For this review, take the finished solid that the model builds, in its own axes (mm). A direction names the side the tool comes from. Give positions to 0.01 mm unless a question says otherwise; leave off trailing zeros. Write each loop counter-clockwise with the first axis right and the second up, starting at its lowest first coordinate (ties: lowest second). Pieces come first, ordered by that corner, then holes. Notation, with made-up numbers: (26.5, -24.5) -> (53.5, -24.5) arc R20 cw to (53.5, -18.5) -> close; hole circle Ø5 at (58, -33). An arc over 180 degrees is marked (long way). Return JSON: item names as keys, results as strings.
from build123d import *

# Parameters (mm, degrees)
CROQUIS2_R            = 2
CORTAR_EXTRUIR1_DEPTH = 10
REDONDEO1_R           = 3


with BuildPart() as part:
    # Croquis1 → Revolución1 (revolve)
    with BuildSketch(Plane.XY, mode=Mode.PRIVATE) as revoluci_n1_sk:
        Polygon((0, 0), (2, 0), (2, 12), (7, 12), (7, 20), (8.25, 20), (8.25, 32.5), (0, 32.5), align=None)
    revolve(revoluci_n1_sk.sketch.rotate(Axis((0, 32.5, 0), (0, -1, 0)), 90), axis=Axis((0, 32.5, 0), (0, -1, 0)))

    # Croquis2 → Cortar-Extruir1 (cut)
    with BuildSketch(Plane(origin=(0, 32.5, 0), x_dir=(1, 0, 0), z_dir=(0, 1, 0))):
        with Locations(Location((0, 0, 0), (0, 0, 270))):
            Circle(CROQUIS2_R)
    extrude(amount=-CORTAR_EXTRUIR1_DEPTH, mode=Mode.SUBTRACT)

    # Redondeo1
    redondeo1_edges = [part.edges().sort_by_distance(p)[0] for p in [
        (0, 32.5, -8.25),
    ]]
    fillet(redondeo1_edges, radius=REDONDEO1_R)


solid = part.part
1. Add section D-D, the plane y = 9.5. State the section outline as (x, z) points.
Results found:
{"outline": "circle Ø4 at (0, 0)"}
2. For pin 1 (4 mm diameter, centred on x = 0.5, y = 20, fed in from +Z); pin 2 (5 mm diameter, centred on y = 23.5, z = -3, fed in from -X); pin 3 (5 mm diameter, centred on y = 20.5, z = 3, fed in from +X); pin 4 (4 mm diameter, centred on y = 17.5, z = -2.5, fed in from +X), all flat-tipped, find the tip position at first contact; note any pin that passes through.
Results found:
{"pin 1": "stops at z = 8.25", "pin 2": "stops at x = -8.23", "pin 3": "stops at x = 8.23", "pin 4": "stops at x = 6.98"}
3. Add section B-B, the plane y = 27. State the section outline as (x, z) points, plus the area to 3 significant figures.
Results found:
{"outline": "circle Ø16.5 at (0, 0); hole circle Ø4 at (0, 0)", "area": "201 mm²"}
4. For faces 1 (the cylindrical face through (6.21, 16.06, 3.23)), 2 (the flat face through (0, 0, 0)), list the 3-axis set-ups (+Z, -Z, +X, -X, +Y, -Y) from which the entire face can be reached by the end or side of a thin tool; tool diameter is ignored.
Results found:
{"face 1": "-Y", "face 2": "+Z, -Z, +X, -X, -Y"}
5. The part is to be moulded in two halves that separate along X. For faces 3 (the cylindrical face through (2, 6, 0)), 4 (the flat face through (0, 22.5, 0)), 5 (the flat face through (-0.1, 32.5, 2.3)), 6 (the cylindrical face through (-2, 28, 0)), say which applies: +X half, -X half, draft (parallel to the pull), parting line (faces both ways), or undercut.
Results found:
{"face 3": "parting line", "face 4": "undercut", "face 5": "draft", "face 6": "undercut"}
6. Add section A-A, the plane z = 0. State the section outline as (x, y) points.
Results found:
{"outline": "(-8.25, 20) -> (-7, 20) -> (-7, 12) -> (-2, 12) -> (-2, 0) -> (2, 0) -> (2, 12) -> (7, 12) -> (7, 20) -> (8.25, 20) -> (8.25, 29.5) arc R3 ccw to (5.25, 32.5) -> (2, 32.5) -> (2, 22.5) -> (-2, 22.5) -> (-2, 32.5) -> (-5.25, 32.5) arc R3 ccw to (-8.25, 29.5) -> close"}
7. To check wall thickness, follow probe 1 along X at (y, z) = (25.5, 0); probe 2 along Y at (x, z) = (-3.25, -3); probe 3 along X at (y, z) = (24.5, 0.75). State the ranges of each line that lie inside material, in increasing order.
Results found:
{"probe 1": "x = -8.25 to -2, 2 to 8.25", "probe 2": "y = 12 to 32.5", "probe 3": "x = -8.22 to -1.85, 1.85 to 8.22"}
8. Add section C-C, the plane x = 0. State the section outline as (y, z) points, plus the area to 3 significant figures.
Results found:
{"outline": "(0, -2) -> (12, -2) -> (12, -7) -> (20, -7) -> (20, -8.25) -> (29.5, -8.25) arc R3 ccw to (32.5, -5.25) -> (32.5, -2) -> (22.5, -2) -> (22.5, 2) -> (32.5, 2) -> (32.5, 5.25) arc R3 ccw to (29.5, 8.25) -> (20, 8.25) -> (20, 7) -> (12, 7) -> (12, 2) -> (0, 2) -> close", "area": "322 mm²"}
